Here's the drawing with two shaded views (mm, measured from the low corner). I have some questions. A direction names the side the tool comes from. Coordinates: 2 decimals unless noted, no trailing zeros. Write each loop counter-clockwise with the first axis right and the second up, starting at its lowest first coordinate (ties: lowest second). Pieces come first, ordered by that corner, then holes. Notation, with made-up numbers: (57.25, 8) -> (111.25, 8) arc R24 cw to (111.25, 26) -> close; hole circle Ø7 at (56.5, -23.75). An arc over 180 degrees is marked (long way). Use a Markdown table: item, result. Add a question column.
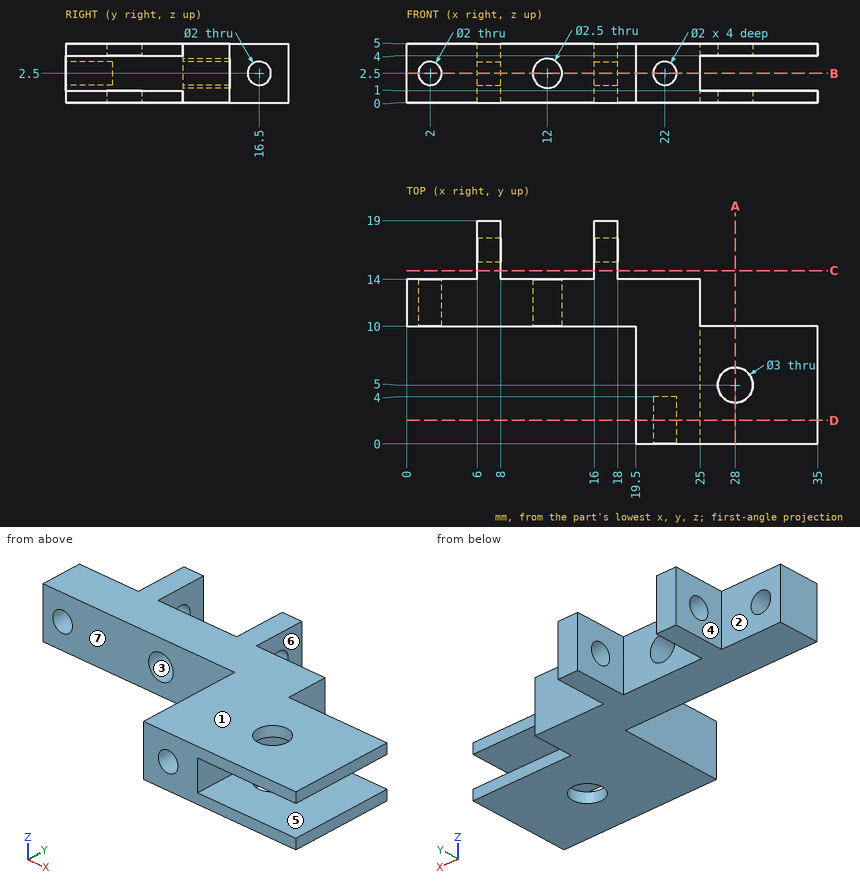
Q1. Please list where these lines run through material, in increasing order: line 1 (Z direction, x = 17.65, y = 16.5); line 2 (X direction, y = 16.25, z = 0.7); line 3 (X direction, y = 5, z = 0.7).
Q2. Suppose I cut it at D-D, the plane y = 2. Write out the boundary of the cut face in (x, z), and give its area (3 significant figures).
Q3. Suppose I cut it at C-C, the plane y = 14.75. Write out the boundary of the cut face in (x, z), and give its area (3 significant figures).
Q4. Suppose I cut it at A-A, the plane x = 28. Write out the boundary of the cut face in (y, z).
Q5. Will these pins go through, and if not, where does the flat tip stop? pin 1 (2.5 mm diameter, centred on y = 2.5, z = 2, fed in from -X); pin 2 (2.5 mm diameter, centred on y = 16.5, z = 2.5, fed in from +X); pin 3 (1.5 mm diameter, centred on x = 2.5, z = 2.5, fed in from +Y); pin 4 (1.8 mm diameter, centred on x = 28, y = 5, fed in from +Z).
Q6. Thinking about a two-plate mould opening in Z: for the marked faces 1, 2 and 3, which applies, released by +Z, released by -Z, zero draft, split by the parting line, or undercut?
Q7. Suppose I cut it at B-B, the plane z = 2.5. State how many separate pieces and enclosed holes the cut face has, and give its area (3 significant figures).
Q8. Which directions (+Z, -Z, +X, -X, +Y, -Y) give clear straight access to the entire face, cutting with the end or side of a thin tool? Please do the marked faces 4, 5, 6 and 7.
Answer key:
| question | item | result |
|---|---|---|
| 1 | line 1 | z = 0 to 1.5, 3.5 to 5 |
| 1 | line 2 | x = 6 to 8, 16 to 18 |
| 1 | line 3 | x = 19.5 to 26.5, 29.5 to 35 |
| 2 | outline | (19.5, 0) -> (35, 0) -> (35, 1) -> (25, 1) -> (25, 4) -> (35, 4) -> (35, 5) -> (19.5, 5) -> close; hole circle Ø2 at (22, 2.5) |
| 2 | area | 44.4 mm^2 |
| 3 | outline | (6, 0) -> (8, 0) -> (8, 5) -> (6, 5) -> close; (16, 0) -> (18, 0) -> (18, 5) -> (16, 5) -> close |
| 3 | area | 20.0 mm^2 |
| 4 | outline | (0, 0) -> (3.5, 0) -> (3.5, 1) -> (0, 1) -> close; (0, 4) -> (3.5, 4) -> (3.5, 5) -> (0, 5) -> close; (6.5, 0) -> (10, 0) -> (10, 1) -> (6.5, 1) -> close; (6.5, 4) -> (10, 4) -> (10, 5) -> (6.5, 5) -> close |
| 5 | pin 1 | stops at x = 19.5 |
| 5 | pin 2 | stops at x = 18 |
| 5 | pin 3 | stops at y = 14 |
| 5 | pin 4 | passes through |
| 6 | face 1 | released by +Z |
| 6 | face 2 | zero draft |
| 6 | face 3 | undercut |
| 7 | separate pieces | 5 |
| 7 | enclosed holes | 0 |
| 7 | area | 141 mm^2 |
| 8 | face 4 | +Z, -Z, -X, +Y |
| 8 | face 5 | +X, +Y, -Y |
| 8 | face 6 | +Z, -Z, +X, +Y |
| 8 | face 7 | +Z, -Z, -X, -Y |
